Here's how the part is built. I have some questions about the finished solid (model axes, mm). Round coordinates to 2 decimals unless told otherwise and drop trailing zeros. Loops run counter-clockwise (first coordinate to the right, second up) from the corner with the lowest first, then second, coordinate; pieces in that order, holes last. Notation, with made-up numbers: M -27,48.5 L 18,48.5 A7 cw 18,61.5 Z; hole C 30.25,44.5 d8. An arc over 180 degrees is marked long. Write item = value, one per line. Start each with the question number.
Autodesk Inventor part; units mm, degrees
ref_plane "YZ Plane" through (0, 0, 0) normal (1, 0, 0) x (0, 1, 0)
ref_plane "XZ Plane" through (0, 0, 0) normal (0, 1, 0) x (-1, 0, 0)
ref_plane "XY Plane" through (0, 0, 0) normal (0, 0, 1) x (1, 0, 0)
sketch "Sketch1" plane through (0, 0, 0) normal (0, 0, 1) x (1, 0, 0)
  line L0 (0, 0) -> (22.225, 0)
  line L1 (22.225, 0) -> (22.225, 25.4)
  line L2 (22.225, 25.4) -> (0, 25.4)
  line L3 (0, 25.4) -> (0, 0)
  arc A0 (22.225, 25.4) -> (0, 25.4) centre (11.1125, 25.4) ccw
  dimension "d0" = 25.4
  dimension "d1" = 22.225
  dimension "d4" = 11.1125
extrude "Extrusion2" add sketch "Sketch1" along normal blind 22.225
sketch "Sketch2" plane through (0, 0, 22.225) normal (0, 0, 1) x (1, 0, 0)
  line L0 (0, 0) -> (22.225, 0)
  line L1 (22.225, 0) -> (22.225, 25.4)
  point P0 (11.1125, 23.8252)
  dimension "d7" = 23.8252
  dimension "d8" = 11.1125
hole "Hole1" at (11.1125, 23.8252, 22.225) direction (0, 0, -1) diameter 6.35 end through all
properties part number "CLB_053_ScissorTopBarPlug" material "Nylon 6/6"
Item 1: Will these pins go through, and if not, where does the flat tip stop? pin 1 Ø1.5 at (x, z) = (18.5, 18) entering from +Y; pin 2 Ø1 at (y, z) = (27, 18.5) entering from -X.
Item 2: I want a section at C-C, the plane x = 3.5. List the corners of the cut face in (y, z) for me (3 decimals).
Item 3: We'd pull the mould along X, two halves only. Please class faces 1 (the flat face through (11, 0, 11)), 2 (the cylindrical face through (8.97, 26.17, 10.96)), 3 (the cylindrical face through (10.87, 36.51, 10.96)): released by +X, released by -X, zero draft, split by the parting line, or undercut.
Item 4: I want a section at B-B, the plane x = 17. List the corners of the cut face in (y, z) for me (3 decimals).
Item 5: Please list where these lines run through material, in increasing order: line 1 (Y direction, x = 12.25, z = 8.25); line 2 (X direction, y = 23.5, z = 8) (3 decimals); line 3 (X direction, y = 26.5, z = 4.25). Write a range as [from, to].
Worked out:
q1.pin_1 = 34.31
q1.pin_2 = 0.05
q2.outline = M 0,0 L 33.496,0 L 33.496,22.225 L 0,22.225 Z
q3.face_1 = zero draft
q3.face_2 = undercut
q3.face_3 = split by the parting line
q4.outline = M 0,0 L 34.825,0 L 34.825,22.225 L 0,22.225 Z
q5.line_1 = [0, 20.86], [26.79, 36.45]
q5.line_2 = [0, 7.954], [14.271, 22.225]
q5.line_3 = [0.05, 9.4], [12.82, 22.17]
